from build123d import *

# Parameters (mm, degrees)
SKETCH1_W           = 104
SKETCH1_H           = 104
BOSS_EXTRUDE1_DEPTH = 115
CUT_EXTRUDE1_DEPTH  = 164.538986178
CUT_EXTRUDE2_DEPTH  = 57.5
SKETCH4_R           = 25
CUT_EXTRUDE3_DEPTH  = 137.502747225
SKETCH5_R           = 35
CUT_EXTRUDE4_DEPTH  = 10
CUT_EXTRUDE5_START  = -10
SKETCH6_R           = 35
CUT_EXTRUDE5_DEPTH  = 10
SKETCH7_W           = 52
SKETCH7_H           = 52
CUT_EXTRUDE6_DEPTH  = 137.502747225
FILLET2_R           = 15
FILLET3_R           = 15
BOSS_EXTRUDE2_DEPTH = 10
CUT_EXTRUDE7_DEPTH  = 10


with BuildPart() as part:
    # Sketch1 → Boss-Extrude1 (new body)
    with BuildSketch(Plane(origin=(0, 0, 0), x_dir=(1, 0, 0), z_dir=(0, 1, 0))):
        Rectangle(SKETCH1_W, SKETCH1_H)
    extrude(amount=BOSS_EXTRUDE1_DEPTH)

    # Sketch2 → Cut-Extrude1 (cut, through all)
    with BuildSketch(Plane(origin=(52, 0, 0), x_dir=(0, 0, -1), z_dir=(1, 0, 0))):
        Polygon((-52, 115), (-52, 0), (-27.592698068, 57.5), align=None)
        Polygon((52, 115), (52, 0), (27.592698068, 57.5), align=None)
    extrude(amount=-CUT_EXTRUDE1_DEPTH, mode=Mode.SUBTRACT)

    # Sketch3 → Cut-Extrude2 (cut, symmetric)
    with BuildSketch(Plane.XY):
        Polygon((-52, 115), (-27.592698068, 57.5), (-52, 0), align=None)
        Polygon((52, 0), (27.592698068, 57.5), (52, 115), align=None)
    extrude(amount=CUT_EXTRUDE2_DEPTH, both=True, mode=Mode.SUBTRACT)

    # Sketch4 → Cut-Extrude3 (cut, through all)
    with BuildSketch(Plane(origin=(0, 115, 0), x_dir=(1, 0, 0), z_dir=(0, 1, 0))):
        with Locations(Location((0, 0, 0), (0, 0, 270))):
            Circle(SKETCH4_R)
    extrude(amount=-CUT_EXTRUDE3_DEPTH, mode=Mode.SUBTRACT)

    # Sketch5 → Cut-Extrude4 (cut)
    with BuildSketch(Plane(origin=(0, 115, 0), x_dir=(1, 0, 0), z_dir=(0, 1, 0))):
        with Locations(Location((0, 0, 0), (0, 0, 270))):
            Circle(SKETCH5_R)
    extrude(amount=-CUT_EXTRUDE4_DEPTH, mode=Mode.SUBTRACT)

    # Sketch6 → Cut-Extrude5 (cut)
    with BuildSketch(Plane.XZ.offset(CUT_EXTRUDE5_START)):
        with Locations(Location((0, 0, 0), (0, 0, 90))):
            Circle(SKETCH6_R)
    extrude(amount=CUT_EXTRUDE5_DEPTH, mode=Mode.SUBTRACT)

    # Sketch7 → Cut-Extrude6 (cut, through all)
    with BuildSketch(Plane(origin=(0, 115, 0), x_dir=(1, 0, 0), z_dir=(0, 1, 0))):
        with Locations((26, -26)):
            Rectangle(SKETCH7_W, SKETCH7_H)
    extrude(amount=-CUT_EXTRUDE6_DEPTH, mode=Mode.SUBTRACT)

    # Fillet2
    fillet2_edges = [part.edges().sort_by_distance(p)[0] for p in [
        (0, 57.5, -27.592698068),
    ]]
    fillet(fillet2_edges, radius=FILLET2_R)

    # Fillet3
    fillet3_edges = [part.edges().sort_by_distance(p)[0] for p in [
        (-13.796349034, 57.5, 27.592698068),
    ]]
    fillet(fillet3_edges, radius=FILLET3_R)

    # Sketch8 → Boss-Extrude2 (add)
    with BuildSketch(Plane(origin=(0, 115, 0), x_dir=(1, 0, 0), z_dir=(0, 1, 0))):
        Polygon((-49, 49), (49, 49), (49, 0), (52, 0), (52, 52), (-52, 52), (-52, -52), (0, -52), (0, -49), (-49, -49), align=None)
    extrude(amount=BOSS_EXTRUDE2_DEPTH)

    # Sketch9 → Cut-Extrude7 (cut)
    with BuildSketch(Plane(origin=(0, 115, 0), x_dir=(1, 0, 0), z_dir=(0, 1, 0))):
        with BuildLine():
            Line((-40.734018716, 44.976659403), (-25.734018716, 29.976659403))
            ThreePointArc((-25.734018716, 29.976659403), (-25.734018716, 25.734018716), (-29.976659403, 25.734018716))
            Line((-29.976659403, 25.734018716), (-44.976659403, 40.734018716))
            ThreePointArc((-44.976659403, 40.734018716), (-44.976659403, 44.976659403), (-40.734018716, 44.976659403))
        make_face()
        with BuildLine():
            Line((44.976659403, 40.734018716), (29.976659403, 25.734018716))
            ThreePointArc((29.976659403, 25.734018716), (25.734018716, 25.734018716), (25.734018716, 29.976659403))
            Line((25.734018716, 29.976659403), (40.734018716, 44.976659403))
            ThreePointArc((40.734018716, 44.976659403), (44.976659403, 44.976659403), (44.976659403, 40.734018716))
        make_face()
        with BuildLine():
            Line((-44.976659403, -40.734018716), (-29.976659403, -25.734018716))
            ThreePointArc((-29.976659403, -25.734018716), (-25.734018716, -25.734018716), (-25.734018716, -29.976659403))
            Line((-25.734018716, -29.976659403), (-40.734018716, -44.976659403))
            ThreePointArc((-40.734018716, -44.976659403), (-44.976659403, -44.976659403), (-44.976659403, -40.734018716))
        make_face()
    extrude(amount=-CUT_EXTRUDE7_DEPTH, mode=Mode.SUBTRACT)


solid = part.part
Work out the finished part from the listing and answer in its coordinate system (mm). A direction names the side the tool comes from. Round coordinates to 2 decimals unless told otherwise and drop trailing zeros. Order: outer loops, then holes, each group sorted by start corner. A loop starts at its lowest first (then second) coordinate and runs counter-clockwise, first axis right, second up. Notation, with made-up numbers: M 74.5,-21 L 83.5,-21 A30 ccw 83.5,4 Z; hole C 30,-14 d2. An arc over 180 degrees is marked long. Put each result on its own line as item: value. Start each with the question number.
Q1. Straight lines are drawn through the part: L1, parallel to Y at x = -13.5, z = 22; L2, parallel to X at y = 119, z = 21; L3, parallel to X at y = 46.5, z = -16.5. For each, find the intervals that lie inside material, in ascending order. Write a range as [from, to].
Q2. Section D-D, the plane z = -12.5 is taken. Write down the section's boundary in (x, y), and give its area (3 significant figures).
Q3. For a pull along Z with two mould halves and no side action, classify faces 4 (the flat face through (1, 120, -52)), 5 (the flat face through (-52, 120, -1)), 6 (the flat face through (-18, 105, -18)) as pulls with the +Z half, pulls with the -Z half, needs draft (parallel to the pull), parting line crosses it, or undercut.
Q4. Flat-ended cylindrical pins translate along their axes: pin 1 (8 mm diameter, centred on y = 90.5, z = 4.5, fed in from -X); pin 2 (8 mm diameter, centred on x = 1, z = -34.5, fed in from +Y); pin 3 (23 mm diameter, centred on x = 39, z = -31, fed in from +Y); pin 4 (5 mm diameter, centred on x = 12, y = 55, fed in from +Z). Find the tip coordinate at first contact, or state that the pin passes through.
Q5. A tool of negligible diameter and unlimited length cuts with its end or side. For faces 1 (the cylindrical face through (-45.02, 110.07, -44.93)), 2 (the flat face through (-39.625, 29.152, -0.728)), 3 (the flat face through (39.625, 85.848, -19.858)), from which of +Z, -Z, +X, -X, +Y, -Y can it reach the whole face along a straight path? Write none if from no direction.
Q6. Section B-B, the plane x = -17.5 is taken. Write down the section's boundary in (y, z), and give its area (3 significant figures).
Q7. Section C-C, the plane y = 37 is taken. Write down the section's boundary in (x, z), and give its area (3 significant figures).
Q8. Section A-A, the plane z = 38.5 is taken. Write down the section's boundary in (x, y).
Findings below:
1. L1: y = [10, 105]
1. L2: x = [-52, -49]
1. L3: x = [-32.26, -18.78], [18.78, 32.26]
2. outline: M -52,0 L -32.69,0 L -32.69,10 L -21.65,10 L -21.65,105 L -32.69,105 L -32.69,115 L -49,115 L -49,125 L -52,125 L -52,115 L -27.59,57.5 Z; M 21.65,10 L 32.69,10 L 32.69,0 L 52,0 L 27.59,57.5 L 52,115 L 52,125 L 49,125 L 49,115 L 32.69,115 L 32.69,105 L 21.65,105 Z
2. area: 3,790 mm^2
3. face 4: pulls with the -Z half
3. face 5: needs draft
3. face 6: undercut
4. pin 1: stops at x = -43.3
4. pin 2: stops at y = 115
4. pin 3: stops at y = 125
4. pin 4: stops at z = -20.37
5. face 1: +Y
5. face 2: +Z, -Z, -X
5. face 3: +Z, -Z, +X
6. outline: M 0,-52 L 51.64,-30.08 A15 cw 63.36,-30.08 L 115,-52 L 125,-52 L 125,-49 L 115,-49 L 115,-30.31 L 105,-30.31 L 105,-17.85 L 10,-17.85 L 10,-30.31 L 0,-30.31 Z; M 0,30.31 L 10,30.31 L 10,17.85 L 105,17.85 L 105,30.31 L 115,30.31 L 115,49 L 125,49 L 125,52 L 115,52 L 63.36,30.08 A15 cw 51.64,30.08 L 0,52 Z
6. area: 4,620 mm^2
7. outline: M -36.29,-36.29 L 36.29,-36.29 L 36.29,0 L 25,0 A25 cw long 0,25 L 0,36.29 L -36.29,36.29 Z
7. area: 2,480 mm^2
8. outline: M -52,0 L 0,0 L 0,31.8 L -38.5,31.8 Z; M -52,115 L -38.5,83.2 L 0,83.2 L 0,115 L -34.26,115 L -34.26,105 L -42.74,105 L -42.74,115 L -49,115 L -49,125 L -52,125 Z
